Here's how the part is built. I have some questions about the finished solid (model axes, mm). A direction names the side the tool comes from. Round coordinates to 2 decimals unless told otherwise and drop trailing zeros. Loops run counter-clockwise (first coordinate to the right, second up) from the corner with the lowest first, then second, coordinate; pieces in that order, holes last. Notation, with made-up numbers: M 88,3.5 L 132,3.5 A6 ccw 132,14.5 Z; hole C 33.25,81 d11. An arc over 180 degrees is marked long. Write each question's results on one line, items separated by ' | '. Start each with the question number.
```python
from build123d import *


with BuildPart() as part:
    # Sketch1 → Revolve1 (revolve)
    with BuildSketch(Plane(origin=(0, 0, 0), x_dir=(0, 0, -1), z_dir=(1, 0, 0))):
        with BuildLine():
            Line((-79.8322, 28.575), (-20.9042, 28.575))
            Line((-20.9042, 28.575), (-19.3802, 30.099))
            Line((-19.3802, 30.099), (-19.3802, 32.0421))
            Line((-19.3802, 32.0421), (-14.3002, 32.0421))
            Line((-14.3002, 32.0421), (-14.3002, 34.671))
            Line((-14.3002, 34.671), (-9.525, 34.671))
            Line((-9.525, 34.671), (-9.525, 32.4739))
            Line((-9.525, 32.4739), (0, 32.4739))
            Line((0, 32.4739), (0, 26.5811))
            Line((0, 26.5811), (-6.195945658, 15.84940732))
            ThreePointArc((-6.195945658, 15.84940732), (-11.462350599, 10.596653993), (-18.654516145, 8.6995))
            Line((-18.654516145, 8.6995), (-23.429716145, 8.6995))
            Line((-23.429716145, 8.6995), (-79.8322, 23.8125))
            Line((-79.8322, 23.8125), (-79.8322, 28.575))
        make_face()
    revolve(axis=Axis((0, 0, 0), (0, 0, 1)))


solid = part.part
```
Item 1: I'm going to push flat-ended pins straight in: pin 1 (6 mm diameter, centred on x = 21, z = 61, fed in from -Y); pin 2 (21 mm diameter, centred on x = 0, y = 4, fed in from -Z); pin 3 (2 mm diameter, centred on x = 8.5, z = 49, fed in from -Y). Where does each tip first touch, or does it pass through?
Item 2: If we section it at C-C on z = 38.5: Please give me the cut outline in (x, y) (3 decimals).
Item 3: If we mould it in two halves opening along Y, with no side actions, what happens to faces 1 (the face through (0, -27, 0)), 2 (the face through (-1.524, -34.637, 11.879)), 3 (the face through (-16.231, -2.131, 5.895))? For each: released by +Y, released by -Y, zero draft, split by the parting line, or undercut.
Item 4: If we section it at A-A on y = 0: Please give me the cut outline in (x, z) (1 decimal).
Item 5: Which directions (+Z, -Z, +X, -X, +Y, -Y) give clear straight access to the entire face, cutting with the end or side of a thin tool? Please do faces 4 (the face through (-31, -10.4, 9.525)), 5 (the face through (8.49, -1.89, 21.08)), 6 (the face through (-1.256, -28.547, 49.956)).
Item 6: I need wall thicknesses on L1, parallel to X at y = 0, z = 21.5 (1 decimal); L2, parallel to Z at x = -5.5, y = -31. Which ranges of each line are inside material? Lowest first, please.
Numbers:
1) pin 1: y = -22.19 | pin 2: z = 7.08 | pin 3: y = -27.57
2) outline: C 0,0 d57.15; hole C 0,0 d25.475
3) face 1: zero draft | face 2: split by the parting line | face 3: undercut
4) outline: M -34.7,9.5 L -32.5,9.5 L -32.5,0 L -26.6,0 L -15.8,6.2 A14.3 ccw -8.7,18.7 L -8.7,23.4 L -23.8,79.8 L -28.6,79.8 L -28.6,20.9 L -30.1,19.4 L -32,19.4 L -32,14.3 L -34.7,14.3 Z; M 8.7,18.7 A14.3 ccw 15.8,6.2 L 26.6,0 L 32.5,0 L 32.5,9.5 L 34.7,9.5 L 34.7,14.3 L 32,14.3 L 32,19.4 L 30.1,19.4 L 28.6,20.9 L 28.6,79.8 L 23.8,79.8 L 8.7,23.4 Z
5) face 4: -Z | face 5: +Z, -Z | face 6: +Z
6) L1: -28.6 to -8.7, 8.7 to 28.6 | L2: 0 to 19.38
